from build123d import *
from build123d.topology import SkipClean

# Parameters (mm, degrees)
SKETCH_1_R          = 26
SKETCH_1_R_2        = 12
SKETCH_1_R_3        = 2
EXTRUDE_1_DEPTH     = 3
SKETCH_2_R          = 18
SKETCH_2_R_2        = 13.9
EXTRUDE_2_DEPTH     = 11
SKETCH_3_R          = 1.5
CUT_EXTRUDE_1_DEPTH = 40.344631146
SKETCH_4_R          = 3
CUT_EXTRUDE_5_DEPTH = 11
EXTRUDE_3_DEPTH     = 3.5


with BuildPart() as part:
    # 草图1 → 凸台-拉伸1 (new body)
    with BuildSketch(Plane.XY):
        Circle(SKETCH_1_R)
        Circle(SKETCH_1_R_2, mode=Mode.SUBTRACT)
        with Locations((-15.556349186, 15.556349186)):
            Circle(SKETCH_1_R_3, mode=Mode.SUBTRACT)
        with Locations((15.556349186, 15.556349186)):
            Circle(SKETCH_1_R_3, mode=Mode.SUBTRACT)
        with Locations((15.556349186, -15.556349186)):
            Circle(SKETCH_1_R_3, mode=Mode.SUBTRACT)
        with Locations((-15.556349186, -15.556349186)):
            Circle(SKETCH_1_R_3, mode=Mode.SUBTRACT)
    extrude(amount=EXTRUDE_1_DEPTH)

    # 草图2 → 凸台-拉伸2 (add)
    with BuildSketch(Plane.XY.offset(3)):
        Circle(SKETCH_2_R)
        Circle(SKETCH_2_R_2, mode=Mode.SUBTRACT)
    extrude(amount=EXTRUDE_2_DEPTH)

    # 草图3 → 切除-拉伸1 (cut, through all)
    with BuildSketch(Plane(origin=(0, 0, 0), x_dir=(-1, 0, 0), z_dir=(0, 0, -1))):
        with Locations((0, 14)):
            Circle(SKETCH_3_R)
        with Locations((14, 0)):
            Circle(SKETCH_3_R)
        with Locations((0, -14)):
            Circle(SKETCH_3_R)
        with Locations((-14, 0)):
            Circle(SKETCH_3_R)
    extrude(amount=-CUT_EXTRUDE_1_DEPTH, mode=Mode.SUBTRACT)

    # 草图4 → 切除-拉伸5 (cut)
    with BuildSketch(Plane.XY.offset(14)):
        with Locations((0, 14)):
            Circle(SKETCH_4_R)
        with Locations((14, 0)):
            Circle(SKETCH_4_R)
        with Locations((0, -14)):
            Circle(SKETCH_4_R)
        with Locations((-14, 0)):
            Circle(SKETCH_4_R)
    extrude(amount=-CUT_EXTRUDE_5_DEPTH, mode=Mode.SUBTRACT)

    # 草图5 → 凸台-拉伸3 (add)
    with SkipClean():  # the faces are left unmerged after this step: merging them gives an invalid solid
        with BuildSketch(Plane.XY.offset(3)):
            with BuildLine():
                ThreePointArc((-13.578928571, -2.970302822), (-12.623202626, -2.665413475), (-11.821428571, -2.062480674))
                ThreePointArc((-11.821428571, -2.062480674), (-8.485281374, -8.485281374), (-2.062480674, -11.821428571))
                ThreePointArc((-2.062480674, -11.821428571), (-2.665413475, -12.623202626), (-2.970302822, -13.578928571))
                ThreePointArc((-2.970302822, -13.578928571), (-9.828784258, -9.828784258), (-13.578928571, -2.970302822))
            make_face()
            with BuildLine():
                ThreePointArc((-2.970302822, 13.578928571), (-2.665413475, 12.623202626), (-2.062480674, 11.821428571))
                ThreePointArc((-2.062480674, 11.821428571), (-8.485281374, 8.485281374), (-11.821428571, 2.062480674))
                ThreePointArc((-11.821428571, 2.062480674), (-12.623202626, 2.665413475), (-13.578928571, 2.970302822))
                ThreePointArc((-13.578928571, 2.970302822), (-9.828784258, 9.828784258), (-2.970302822, 13.578928571))
            make_face()
            with BuildLine():
                ThreePointArc((13.578928571, 2.970302822), (12.623202626, 2.665413475), (11.821428571, 2.062480674))
                ThreePointArc((11.821428571, 2.062480674), (8.485281374, 8.485281374), (2.062480674, 11.821428571))
                ThreePointArc((2.062480674, 11.821428571), (2.665413475, 12.623202626), (2.970302822, 13.578928571))
                ThreePointArc((2.970302822, 13.578928571), (9.828784258, 9.828784258), (13.578928571, 2.970302822))
            make_face()
            with BuildLine():
                ThreePointArc((2.970302822, -13.578928571), (2.665413475, -12.623202626), (2.062480674, -11.821428571))
                ThreePointArc((2.062480674, -11.821428571), (8.485281374, -8.485281374), (11.821428571, -2.062480674))
                ThreePointArc((11.821428571, -2.062480674), (12.623202626, -2.665413475), (13.578928571, -2.970302822))
                ThreePointArc((13.578928571, -2.970302822), (9.828784258, -9.828784258), (2.970302822, -13.578928571))
            make_face()
        extrude(amount=EXTRUDE_3_DEPTH)


solid = part.part
Input: part model. Units: mm. Frame: model coordinates. A direction names the side the tool comes from. Round coordinates to 2 decimals unless told otherwise and drop trailing zeros. Write each loop counter-clockwise with the first axis right and the second up, starting at its lowest first coordinate (ties: lowest second). Pieces come first, ordered by that corner, then holes.
1) Reachability of faces 4 (the flat face through (-9, 9, 6.5)), 5 (the cylindrical face through (14, 14.3, 1.5)) from +Z, -Z, +X, -X, +Y, -Y: full face, straight path, thin tool, end or side. Return the list, or none.
2) Draft query along X for faces 1 (the cylindrical face through (-17.554, 15.644, 1.479)), 2 (the flat face through (11, -9, 14)), 3 (the cylindrical face through (-20.633, -15.821, 1.479)). Return one class per face: pulls with the +X half, pulls with the -X half, needs draft (parallel to the pull), parting line crosses it, or undercut.
3) Ray query, L1, parallel to Y at x = 0, z = 7.5; L2, parallel to Z at x = -18.5, y = 13.5; L3, parallel to X at y = 6, z = 4.25. Return the intervals inside material, ascending.
4) Cut plane D-D (y = -9.5). Return the cut outline in (x, z).
5) Contact query for flat-ended pins moving along their axis: P1, Ø4, axis at x = -0.5, y = 13.5, coming from the +Z side; P2, Ø3, axis at x = 15.56, y = -15.56, coming from the -Z side; P3, Ø5, axis at x = 8.5, z = 9, coming from the -Y side; P4, Ø2, axis at y = 17, z = 7, coming from the -X side. Output: stop coordinate, or through.
6) Cut plane A-A (x = 0). Return the cut outline in (y, z).
7) Cut plane C-C (z = 12). Return the cut outline in (x, y).
Geometry says:
1. face 4: +Z
1. face 5: +Z, -Z
2. face 1: undercut
2. face 2: needs draft
2. face 3: parting line crosses it
3. L1: y = -18 to -17, 17 to 18
3. L2: z = 0 to 3
3. L3: x = -16.97 to -10.39, 10.39 to 16.97
4. outline: (-24.2, 0) - (-7.33, 0) - (-7.33, 6.5) - (-10.15, 6.5) - (-10.15, 14) - (-15.29, 14) - (-15.29, 3) - (-24.2, 3) - close; (7.33, 0) - (24.2, 0) - (24.2, 3) - (15.29, 3) - (15.29, 14) - (10.15, 14) - (10.15, 6.5) - (7.33, 6.5) - close
5. P1: stops at z = 3
5. P2: passes through
5. P3: stops at y = -16.97
5. P4: stops at x = -8.25
6. outline: (-26, 0) - (-15.5, 0) - (-15.5, 3) - (-17, 3) - (-17, 14) - (-18, 14) - (-18, 3) - (-26, 3) - close; (-12.5, 0) - (-12, 0) - (-12, 3) - (-12.5, 3) - close; (12, 0) - (12.5, 0) - (12.5, 3) - (12, 3) - close; (15.5, 0) - (26, 0) - (26, 3) - (18, 3) - (18, 14) - (17, 14) - (17, 3) - (15.5, 3) - close
7. outline: circle Ø36 at (0, 0); hole (-13.58, -2.97) arc R13.9 ccw to (-2.97, -13.58) arc R3 ccw (long way) to (2.97, -13.58) arc R13.9 ccw to (13.58, -2.97) arc R3 ccw (long way) to (13.58, 2.97) arc R13.9 ccw to (2.97, 13.58) arc R3 ccw (long way) to (-2.97, 13.58) arc R13.9 ccw to (-13.58, 2.97) arc R3 ccw (long way) to start
